Answer from the drawing. Dimensions are ordinates in mm from the lowest x, y and z of the part. Give positions to 0.01 mm unless a question says otherwise; leave off trailing zeros. Write each loop counter-clockwise with the first axis right and the second up, starting at its lowest first coordinate (ties: lowest second). Pieces come first, ordered by that corner, then holes. Notation, with made-up numbers: M 50.25,-14.75 L 105.25,-14.75 A20 cw 105.25,16.25 Z; hole C -22.75,-29.5 d5. An arc over 180 degrees is marked long. Answer as a JSON object with one key per item and string values.
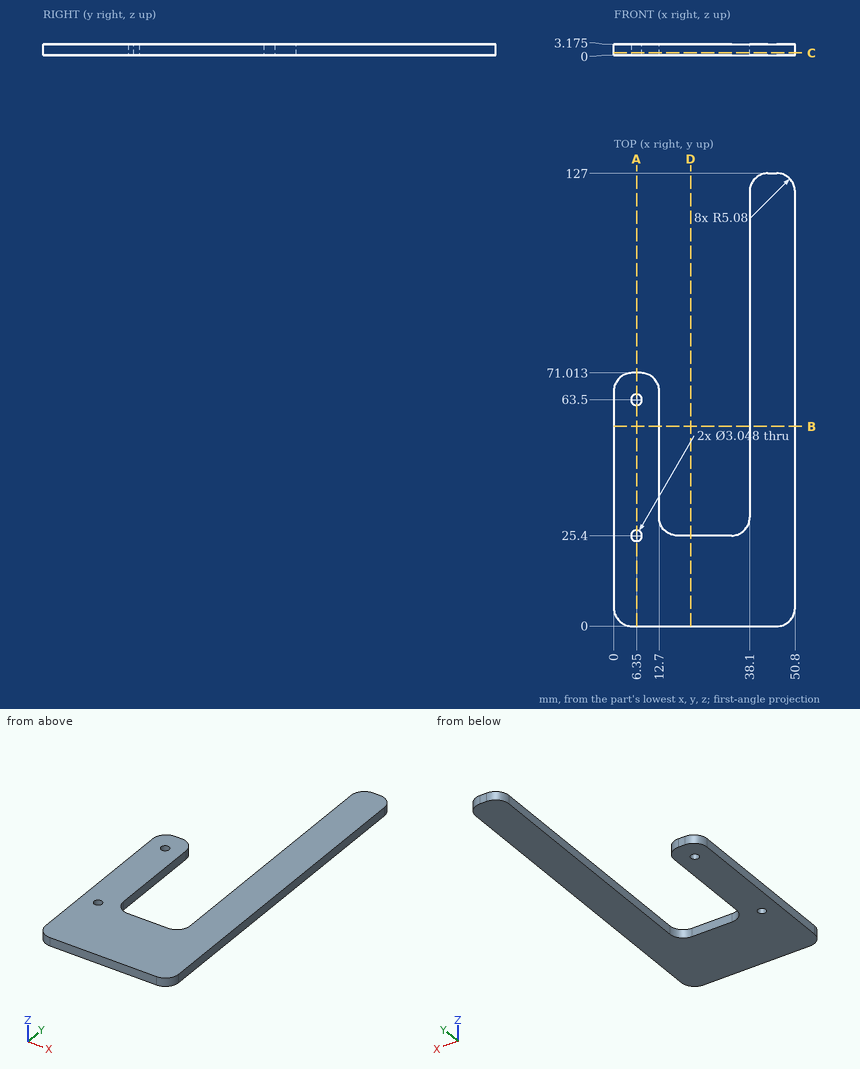
1. Consider line 1 along Y through (x, z) = (6.35, 1.5); line 2 along X through (y, z) = (61, 1.2); line 3 along Y through (x, z) = (30.5, 1.05). Determine where each line is inside the solid, lowest interval first.
Verdict:
{"line 1": "y = 0 to 23.88, 26.92 to 61.98, 65.02 to 71.01", "line 2": "x = 0 to 12.7, 38.1 to 50.8", "line 3": "y = 0 to 25.4"}
2. A flat-ended cylindrical pin translates along its axis: pin 1 (5 mm diameter, centred on x = 6.35, y = 63.5, fed in from +Z) (3 decimals). Find the tip coordinate at first contact, or state that the pin passes through.
Verdict:
{"pin 1": "stops at z = 3.175"}
3. A cutting plane is placed at D-D, the plane x = 21.5. Give the vertices of the cut face in (y, z) (3 decimals).
Verdict:
{"outline": "M 0,0 L 25.4,0 L 25.4,3.175 L 0,3.175 Z"}
4. A cutting plane is placed at B-B, the plane y = 56. Give the vertices of the cut face in (x, z) (3 decimals).
Verdict:
{"outline": "M 0,0 L 12.7,0 L 12.7,3.175 L 0,3.175 Z; M 38.1,0 L 50.8,0 L 50.8,3.175 L 38.1,3.175 Z"}
5. A cutting plane is placed at A-A, the plane x = 6.35. Give the vertices of the cut face in (y, z) (3 decimals), plus the area to 3 significant figures.
Verdict:
{"outline": "M 0,0 L 23.876,0 L 23.876,3.175 L 0,3.175 Z; M 26.924,0 L 61.976,0 L 61.976,3.175 L 26.924,3.175 Z; M 65.024,0 L 71.013,0 L 71.013,3.175 L 65.024,3.175 Z", "area": "206 mm2"}
6. A cutting plane is placed at C-C, the plane z = 0.7. Give the vertices of the cut face in (x, y), plus the area to 3 significant figures.
Verdict:
{"outline": "M 0,5.08 A5.08 ccw 5.08,0 L 45.72,0 A5.08 ccw 50.8,5.08 L 50.8,121.92 A5.08 ccw 45.72,127 L 43.18,127 A5.08 ccw 38.1,121.92 L 38.1,30.48 A5.08 cw 33.02,25.4 L 17.78,25.4 A5.08 cw 12.7,30.48 L 12.7,65.93 A5.08 ccw 7.62,71.01 L 5.08,71.01 A5.08 ccw 0,65.93 Z; hole C 6.35,25.4 d3.05; hole C 6.35,63.5 d3.05", "area": "3,120 mm2"}
